from build123d import *

# Parameters (mm, degrees)
F1_DEPTH = 2


with BuildPart() as f1:
    # F0 (on Top) → F1 (new body)
    with BuildSketch(Plane.XY):
        with BuildLine():
            ThreePointArc((100, -55.5), (98.535534, -59.035534), (95, -60.5))
            Line((95, -60.5), (-13, -60.5))
            Line((-13, -60.5), (-13, -62.5))
            Line((-13, -62.5), (97, -62.5))
            ThreePointArc((97, -62.5), (100.535534, -61.035534), (102, -57.5))
            Line((102, -57.5), (102, 31.5))
            ThreePointArc((102, 31.5), (100.535534, 35.035534), (97, 36.5))
            Line((97, 36.5), (-13, 36.5))
            Line((-13, 36.5), (-13, 34.5))
            Line((-13, 34.5), (95, 34.5))
            ThreePointArc((95, 34.5), (98.535534, 33.035534), (100, 29.5))
            Line((100, 29.5), (100, -55.5))
        make_face()
    extrude(amount=F1_DEPTH)


solid = f1.part
Can you work these out from the model? Positions are in its coordinate system, mm. A direction names the side the tool comes from. Give positions to 0.01 mm unless a question says otherwise; leave off trailing zeros. Order: outer loops, then holes, each group sorted by start corner. A loop starts at its lowest first (then second) coordinate and runs counter-clockwise, first axis right, second up. Notation, with made-up numbers: M 75,29.5 L 120,29.5 A30 ccw 120,66.5 Z; hole C 10,-16 d10. An arc over 180 degrees is marked long. Use one line per item in the form item = value. Start each with the question number.
Item 1: Will this pin go through, and if not, where does the flat tip stop? pin 1 Ø1 at (y, z) = (-15.5, 1) entering from -X.
Item 2: If I drill on line 1 along Y through (x, z) = (-3, 1.15); line 2 along X through (y, z) = (-8.5, 0.9), over which ranges is the centre line in solid material (lowest first)?
Item 3: If we section it at A-A (x = 71.5): Write out the boundary of the cut face in (y, z), then the cut area to 3 significant figures.
Item 4: If we section it at C-C (y = 15.5): Write out the boundary of the cut face in (x, z), then the cut area to 3 significant figures.
Item 5: If we section it at B-B (z = 0.45): Write out the boundary of the cut face in (x, y).
Item 6: We'd pull the mould along Y, two halves only. Please class faces 3 (the cylindrical face through (100.5, -61.07, 0.99)), 4 (the cylindrical face through (100.57, 35, 0.99)), 5 (the cylindrical face through (98.5, 33.07, 0.99)): +Y half, -Y half, draft (parallel to the pull), parting line (faces both ways), or undercut.
Item 7: For faces 1 (the cylindrical face through (98.57, -59, 0.99)), 2 (the flat face through (44, 35, 0)), which set-ups out of +Z, -Z, +X, -X, +Y, -Y let a thin tool reach every point of the face, with its end or its side?
Outcome:
q1.pin_1 = 100
q2.line_1 = -62.5 to -60.5, 34.5 to 36.5
q2.line_2 = 100 to 102
q3.outline = M -62.5,0 L -60.5,0 L -60.5,2 L -62.5,2 Z; M 34.5,0 L 36.5,0 L 36.5,2 L 34.5,2 Z
q3.area = 8.00 mm2
q4.outline = M 100,0 L 102,0 L 102,2 L 100,2 Z
q4.area = 4.00 mm2
q5.outline = M -13,-62.5 L 97,-62.5 A5 ccw 102,-57.5 L 102,31.5 A5 ccw 97,36.5 L -13,36.5 L -13,34.5 L 95,34.5 A5 cw 100,29.5 L 100,-55.5 A5 cw 95,-60.5 L -13,-60.5 Z
q6.face_3 = -Y half
q6.face_4 = +Y half
q6.face_5 = undercut
q7.face_1 = +Z, -Z, -X
q7.face_2 = -Z, +X, -X, +Y, -Y
